Part model, mm, in its own coordinate system. Face numbers are marked on the shaded views. Round coordinates to 2 decimals unless told otherwise and drop trailing zeros. Loops run counter-clockwise (first coordinate to the right, second up) from the corner with the lowest first, then second, coordinate; pieces in that order, holes last. Notation, with made-up numbers: (-34, 6.5) - (-16, 6.5) arc R21 cw to (-16, 40.5) - close; hole circle Ø7 at (50.5, 8). An arc over 180 degrees is marked (long way). Put each result on its own line as item: value.
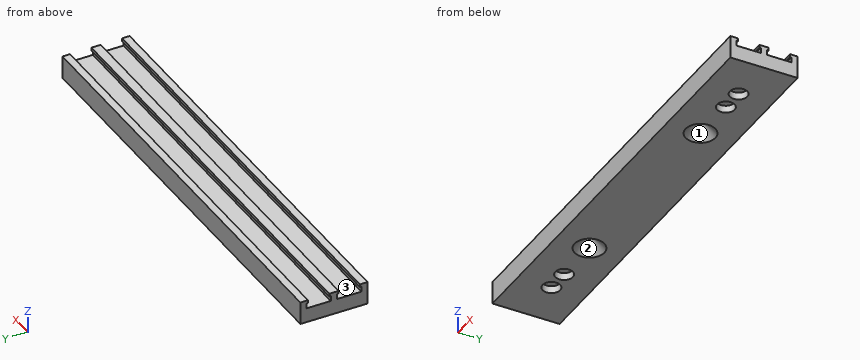
from build123d import *

# Parameters (mm, degrees)
BOX017_W          = 150
BOX017_H          = 7.3
BOX017_DEPTH      = 1
BOX018_W          = 150
BOX018_H          = 7.3
BOX018_DEPTH      = 1
BOX016_W          = 150
BOX016_H          = 8.3
BOX016_DEPTH      = 1.8
BOX015_W          = 150
BOX015_H          = 8.3
BOX015_DEPTH      = 1.8
BOX014_W          = 150
BOX014_H          = 23
BOX014_DEPTH      = 2.8
CYLINDER006_R     = 3
CYLINDER006_DEPTH = 2.5
CYLINDER005_R     = 3
CYLINDER005_DEPTH = 2.5
CYLINDER007_R     = 3
CYLINDER007_DEPTH = 2.5
CYLINDER004_R     = 3
CYLINDER004_DEPTH = 2.5
BOX001_W          = 150
BOX001_H          = 23
BOX001_DEPTH      = 5


with BuildPart() as box017:
    # Box017 → Box017 (new body)
    with BuildSketch(Plane(origin=(0, 2.6, 10.8), x_dir=(1, 0, 0), z_dir=(0, 0, 1))):
        with Locations((75, 3.65)):
            Rectangle(BOX017_W, BOX017_H)
    extrude(amount=BOX017_DEPTH)


with BuildPart() as box018:
    # Box018 → Box018 (new body)
    with BuildSketch(Plane(origin=(0, 13.1, 10.8), x_dir=(1, 0, 0), z_dir=(0, 0, 1))):
        with Locations((75, 3.65)):
            Rectangle(BOX018_W, BOX018_H)
    extrude(amount=BOX018_DEPTH)


with BuildPart() as box016:
    # Box016 → Box016 (new body)
    with BuildSketch(Plane(origin=(0, 12.6, 9), x_dir=(1, 0, 0), z_dir=(0, 0, 1))):
        with Locations((75, 4.15)):
            Rectangle(BOX016_W, BOX016_H)
    extrude(amount=BOX016_DEPTH)


with BuildPart() as fusion006:
    # Box015 → Box015 (new body)
    with BuildSketch(Plane(origin=(0, 2.1, 9), x_dir=(1, 0, 0), z_dir=(0, 0, 1))):
        with Locations((75, 4.15)):
            Rectangle(BOX015_W, BOX015_H)
    extrude(amount=BOX015_DEPTH)

    # Fusion006: union Box017, Box018, Box016
    add(box017.part)
    add(box018.part)
    add(box016.part)


with BuildPart() as f_2x_8mm_tape:
    # Box014 → Box014 (new body)
    with BuildSketch(Plane.XY.offset(9)):
        with Locations((75, 11.5)):
            Rectangle(BOX014_W, BOX014_H)
    extrude(amount=BOX014_DEPTH)

    # Cut006: cut Fusion006
    add(fusion006.part, mode=Mode.SUBTRACT)


with BuildPart() as f_2x_8mm_tape_1:
    # Cut006 placement: moved
    add(f_2x_8mm_tape.part.moved(Location((0, 0, -1))))


with BuildPart() as cone002:
    # Cone002 → Cone002 (revolve)
    with BuildSketch(Plane(origin=(40, 11.5, 3), x_dir=(1, 0, 0), z_dir=(0, -1, 0))):
        Polygon((0, 0), (5.1, 0), (1.1, 4.1), (0, 4.1), align=None)
    revolve(axis=Axis((40, 11.5, 3), (0, 0, 1)))


with BuildPart() as cone003:
    # Cone003 → Cone003 (revolve)
    with BuildSketch(Plane(origin=(110, 11.5, 3), x_dir=(1, 0, 0), z_dir=(0, -1, 0))):
        Polygon((0, 0), (5.1, 0), (1.1, 4.1), (0, 4.1), align=None)
    revolve(axis=Axis((110, 11.5, 3), (0, 0, 1)))


with BuildPart() as cylinder006:
    # Cylinder006 → Cylinder006 (new body)
    with BuildSketch(Plane(origin=(24, 11.5, 3), x_dir=(1, 0, 0), z_dir=(0, 0, 1))):
        Circle(CYLINDER006_R)
    extrude(amount=CYLINDER006_DEPTH)


with BuildPart() as cylinder005:
    # Cylinder005 → Cylinder005 (new body)
    with BuildSketch(Plane(origin=(126, 11.5, 3), x_dir=(1, 0, 0), z_dir=(0, 0, 1))):
        Circle(CYLINDER005_R)
    extrude(amount=CYLINDER005_DEPTH)


with BuildPart() as cylinder007:
    # Cylinder007 → Cylinder007 (new body)
    with BuildSketch(Plane(origin=(134, 11.5, 3), x_dir=(1, 0, 0), z_dir=(0, 0, 1))):
        Circle(CYLINDER007_R)
    extrude(amount=CYLINDER007_DEPTH)


with BuildPart() as removals:
    # Cylinder004 → Cylinder004 (new body)
    with BuildSketch(Plane(origin=(16, 11.5, 3), x_dir=(1, 0, 0), z_dir=(0, 0, 1))):
        Circle(CYLINDER004_R)
    extrude(amount=CYLINDER004_DEPTH)

    # Fusion002: union Cone002, Cone003, Cylinder006, Cylinder005, Cylinder007
    add(cone002.part)
    add(cone003.part)
    add(cylinder006.part)
    add(cylinder005.part)
    add(cylinder007.part)


with BuildPart() as top_2x_8mm:
    # Box001 → Box001 (new body)
    with BuildSketch(Plane.XY.offset(3)):
        with Locations((75, 11.5)):
            Rectangle(BOX001_W, BOX001_H)
    extrude(amount=BOX001_DEPTH)

    # Cut001: cut removals
    add(removals.part, mode=Mode.SUBTRACT)

    # Fusion009: union 2X_8mm_tape
    add(f_2x_8mm_tape_1.part)


solid = top_2x_8mm.part
1. Pin check, flat tips, straight feed: P1, Ø9, axis at x = 63.5, y = 18.5, coming from the +Z side; P2, Ø5, axis at x = 24, y = 11.5, coming from the -Z side; P3, Ø2.5, axis at x = 40.5, y = 5, coming from the +Z side; P4, Ø1.1, axis at x = 40.5, y = 11, coming from the -Z side. Stop position of each tip, or through.
A:
P1: stops at z = 10.8
P2: stops at z = 5.5
P3: stops at z = 8
P4: stops at z = 6.94
2. Band-saw the part on B-B (x = 16). List the corners of the cut face in (y, z), plus the area to 3 significant figures.
A:
outline: (0, 3) - (8.5, 3) - (8.5, 5.5) - (14.5, 5.5) - (14.5, 3) - (23, 3) - (23, 10.8) - (20.4, 10.8) - (20.4, 9.8) - (20.9, 9.8) - (20.9, 8) - (12.6, 8) - (12.6, 9.8) - (13.1, 9.8) - (13.1, 10.8) - (9.9, 10.8) - (9.9, 9.8) - (10.4, 9.8) - (10.4, 8) - (2.1, 8) - (2.1, 9.8) - (2.6, 9.8) - (2.6, 10.8) - (0, 10.8) - close
area: 120 mm²
3. Probe line 1 along Y through (x, z) = (35.5, 9.5); line 2 along Z through (x, y) = (141, 20.75); line 3 along Y through (x, z) = (117, 10.25). List the from-to ranges inside material, lowest first. Write a range as [from, to].
A:
line 1: y = [0, 2.1], [10.4, 12.6], [20.9, 23]
line 2: z = [3, 8], [9.8, 10.8]
line 3: y = [0, 2.6], [9.9, 13.1], [20.4, 23]
4. Band-saw the part on A-A (x = 103). List the corners of the cut face in (y, z), plus the area to 3 significant figures.
A:
outline: (0, 3) - (23, 3) - (23, 10.8) - (20.4, 10.8) - (20.4, 9.8) - (20.9, 9.8) - (20.9, 8) - (12.6, 8) - (12.6, 9.8) - (13.1, 9.8) - (13.1, 10.8) - (9.9, 10.8) - (9.9, 9.8) - (10.4, 9.8) - (10.4, 8) - (2.1, 8) - (2.1, 9.8) - (2.6, 9.8) - (2.6, 10.8) - (0, 10.8) - close
area: 135 mm²
5. Two-plate mould, pull along X, no slides. Class the marked faces 1, 2 and 3: pulls with the +X half, pulls with the -X half, needs draft (parallel to the pull), parting line crosses it, or undercut.
A:
face 1: undercut
face 2: undercut
face 3: needs draft
